Autodesk Inventor part; units mm, degrees
ref_plane "YZ Plane" through (0, 0, 0) normal (1, 0, 0) x (0, 1, 0)
ref_plane "XZ Plane" through (0, 0, 0) normal (0, 1, 0) x (-1, 0, 0)
ref_plane "XY Plane" through (0, 0, 0) normal (0, 0, 1) x (1, 0, 0)
sketch "Sketch1" plane through (0, 0, 0) normal (0, 0, 1) x (1, 0, 0)
  circle A0 centre (-7.7782, 0) radius 1.1 construction
  circle A1 centre (7.7782, 0) radius 1.1 construction
  circle A2 centre (0, -7.7782) radius 1.1 construction
  circle A3 centre (0, 7.7782) radius 1.1 construction
  arc A4 (0, 10) -> (-2.698, 9.6292) centre (0, 0) ccw construction
  arc A5 (-2.698, 9.6292) -> (-5.1958, 8.5442) centre (0, 0) ccw construction
  arc A6 (-5.1958, 8.5442) -> (-7.3084, 6.8255) centre (0, 0) ccw construction
  arc A7 (-7.3084, 6.8255) -> (-8.8789, 4.6007) centre (0, 0) ccw construction
  arc A8 (-8.8789, 4.6007) -> (-9.7908, 2.0346) centre (0, 0) ccw construction
  arc A9 (-9.7908, 2.0346) -> (-9.9767, -0.6824) centre (0, 0) ccw construction
  arc A10 (-9.9767, -0.6824) -> (-9.4226, -3.3488) centre (0, 0) ccw construction
  arc A11 (-9.4226, -3.3488) -> (-8.1697, -5.7668) centre (0, 0) ccw construction
  arc A12 (-8.1697, -5.7668) -> (-6.3109, -7.7571) centre (0, 0) ccw construction
  arc A13 (-6.3109, -7.7571) -> (-3.984, -9.1721) centre (0, 0) ccw construction
  arc A14 (-3.984, -9.1721) -> (-1.3617, -9.9069) centre (0, 0) ccw construction
  arc A15 (-1.3617, -9.9069) -> (1.3617, -9.9069) centre (0, 0) ccw construction
  arc A16 (1.3617, -9.9069) -> (3.984, -9.1721) centre (0, 0) ccw construction
  arc A17 (3.984, -9.1721) -> (6.3109, -7.7571) centre (0, 0) ccw construction
  arc A18 (6.3109, -7.7571) -> (8.1697, -5.7668) centre (0, 0) ccw construction
  arc A19 (8.1697, -5.7668) -> (9.4226, -3.3488) centre (0, 0) ccw construction
  arc A20 (9.4226, -3.3488) -> (9.9767, -0.6824) centre (0, 0) ccw construction
  arc A21 (9.9767, -0.6824) -> (9.7908, 2.0346) centre (0, 0) ccw construction
  arc A22 (9.7908, 2.0346) -> (8.8789, 4.6007) centre (0, 0) ccw construction
  arc A23 (8.8789, 4.6007) -> (7.3084, 6.8255) centre (0, 0) ccw construction
  arc A24 (7.3084, 6.8255) -> (5.1958, 8.5442) centre (0, 0) ccw construction
  arc A25 (5.1958, 8.5442) -> (2.698, 9.6292) centre (0, 0) ccw construction
  arc A26 (2.698, 9.6292) -> (0, 10) centre (0, 0) ccw construction
  circle A27 centre (0, 0) radius 9.4226
  circle A28 centre (7.7782, 0) radius 0.9
  circle A29 centre (0, -7.7782) radius 0.9
  circle A30 centre (-7.7782, 0) radius 0.9
  circle A31 centre (0, 7.7782) radius 0.9
  line L0 (-3.5, -3.5) -> (3.5, -3.5)
  line L1 (3.5, -3.5) -> (3.5, 3.5)
  line L2 (3.5, 3.5) -> (-3.5, 3.5)
  line L3 (-3.5, 3.5) -> (-3.5, -3.5)
  line L4 (-3.5, -3.5) -> (3.5, 3.5) construction
  line L5 (3.5, -3.5) -> (-3.5, 3.5) construction
  line L6 (5.25, 5.25) -> (5.25, -5.25)
  line L7 (5.25, -5.25) -> (-5.25, -5.25)
  line L8 (-5.25, -5.25) -> (-5.25, 5.25)
  line L9 (-5.25, 5.25) -> (5.25, 5.25)
  dimension "d0" = 0.2
  dimension "d1" = 0.2
  dimension "d2" = 0.2
  dimension "d3" = 0.2
  dimension "d4" = 7
  dimension "d5" = 7
extrude "Extrusion1" add sketch "Sketch1" along normal blind 0.5 contours A27 | L6 L7 L8 L9
sketch "Sketch2" plane through (0, 0, 0.5) normal (0, 0, 1) x (1, 0, 0)
  line L0 (-3.5, -3.5) -> (-3.5, 3.5)
  line L1 (-3.5, 3.5) -> (3.5, 3.5)
  line L2 (3.5, 3.5) -> (3.5, -3.5)
  line L3 (3.5, -3.5) -> (-3.5, -3.5)
  circle A0 centre (0, 7.7782) radius 0.9
  circle A1 centre (-7.7782, 0) radius 0.9
  circle A2 centre (0, -7.7782) radius 0.9
  circle A3 centre (7.7782, 0) radius 0.9
  circle A4 centre (0, 0) radius 9.4226
extrude "Extrusion2" add sketch "Sketch2" against normal blind 1.5 contours A0 | A1 | A2 | A3
properties part number "200_Lambdaplatte_2_conterplate"
Geometry check sheet. Reference: the model listing, model coordinates, mm. A direction names the side the tool comes from. Coordinates: 2 decimals unless noted, no trailing zeros. Order: outer loops, then holes, each group sorted by start corner. A loop starts at its lowest first (then second) coordinate and runs counter-clockwise, first axis right, second up. Notation, with made-up numbers: M 50.5,32 L 96.5,32 A8 cw 96.5,47 Z; hole C 30,-25 d4. An arc over 180 degrees is marked long. Answer as a JSON object with one key per item and string values.
Q1. Scan lines: line 1 (Z direction, x = -3.75, y = -5.75); line 2 (X direction, y = -0.5, z = 0.05); line 3 (X direction, y = -7.25, z = -0.35). Record each from-to range of solid material in increasing order.
Results are:
{"line 1": "z = 0 to 0.5", "line 2": "x = -9.41 to -3.5, 3.5 to 9.41", "line 3": "x = -0.73 to 0.73"}
Q2. Cross-section at A-A on x = 0. Record the cut outline in (y, z), and give its area (3 significant figures).
Results are:
{"outline": "M -9.42,0 L -8.68,0 L -8.68,-1 L -6.88,-1 L -6.88,0 L -3.5,0 L -3.5,0.5 L -9.42,0.5 Z; M 3.5,0 L 6.88,0 L 6.88,-1 L 8.68,-1 L 8.68,0 L 9.42,0 L 9.42,0.5 L 3.5,0.5 Z", "area": "9.52 mm²"}
Q3. Release check for a two-part mould opening along X. For faces 1 (the cylindrical face through (-0.195, -8.657, -0.493)), 2 (the cylindrical face through (-8.677, 0.04, -0.493)), 3 (the flat face through (0, 8, -1)) record: released by +X, released by -X, zero draft, split by the parting line, or undercut.
Results are:
{"face 1": "split by the parting line", "face 2": "undercut", "face 3": "zero draft"}
Q4. Depth check by flat-ended pin: pin 1 Ø6 at (x, y) = (5.5, -7.5) entering from -Z. Enter the tip coordinate at first touch or a pass-through.
Results are:
{"pin 1": "stops at z = 0"}
Q5. Cross-section at C-C on x = 8. Record the cut outline in (y, z), and give its area (3 significant figures).
Results are:
{"outline": "M -4.98,0 L -0.87,0 L -0.87,-1 L 0.87,-1 L 0.87,0 L 4.98,0 L 4.98,0.5 L -4.98,0.5 Z", "area": "6.72 mm²"}
Q6. Cross-section at D-D on z = -0.3. Record the cut outline in (x, y).
Results are:
{"outline": "C -7.78,0 d1.8; C 0,-7.78 d1.8; C 0,7.78 d1.8; C 7.78,0 d1.8"}
Q7. Tool access check on faces 4 (the flat face through (4, 0, 0)), 5 (the flat face through (0, -8, -1)). Record the directions out of +Z, -Z, +X, -X, +Y, -Y that give a thin tool (end or side, any length) a straight path to the whole face; none if there is none.
Results are:
{"face 4": "-Z", "face 5": "-Z, +X, -X, +Y, -Y"}
